The drawing under review shows one solid part. Ordinate dimensions are in mm from its lowest x, y, z. A direction names the side the tool comes from. Coordinates: 2 decimals unless noted, no trailing zeros. Order: outer loops, then holes, each group sorted by start corner. A loop starts at its lowest first (then second) coordinate and runs counter-clockwise, first axis right, second up. Notation, with made-up numbers: (64, 36.5) -> (78, 36.5) arc R16 cw to (78, 41.5) -> close; hole circle Ø3 at (-19, 86.5). An arc over 180 degrees is marked (long way). Write item = value, one per line.
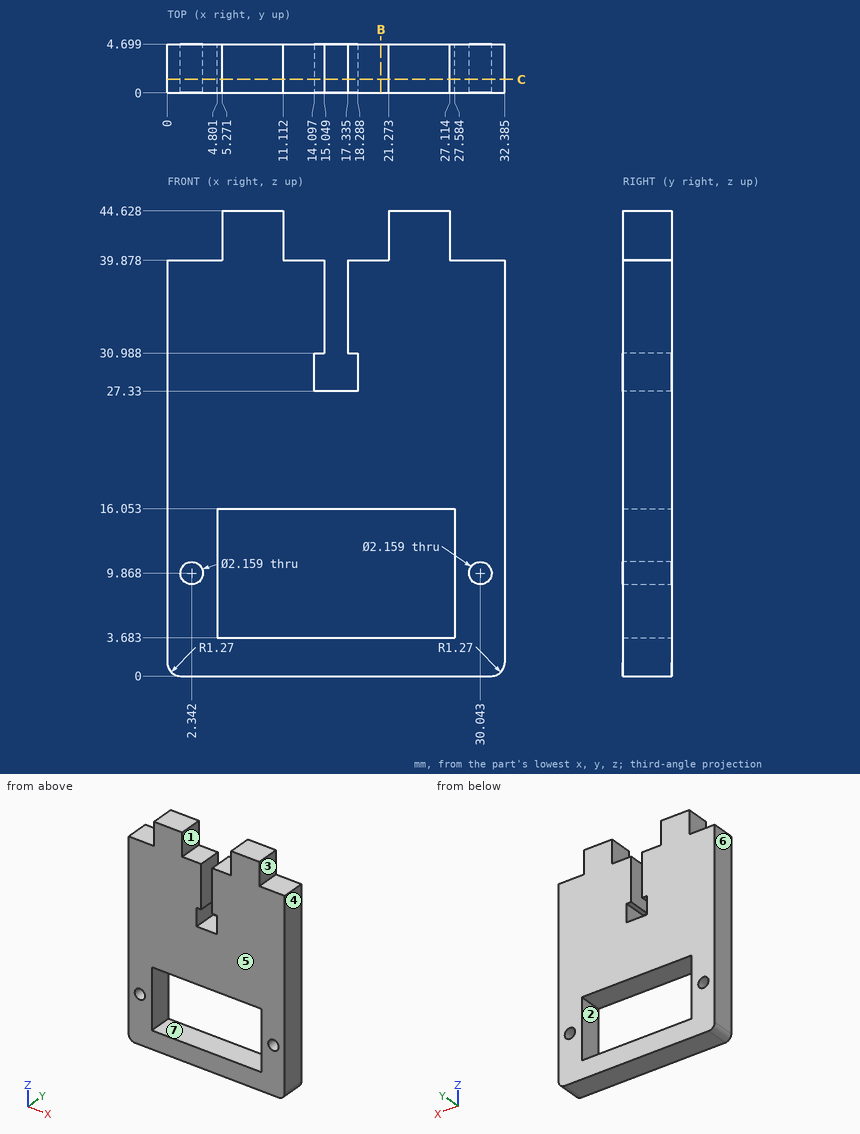
(1) For the marked faces 1, 2, 3 and 4, list the 3-axis set-ups (+Z, -Z, +X, -X, +Y, -Y) from which the entire face can be reached by the end or side of a thin tool; tool diameter is ignored.
Report:
face_1 = +Z, +Y, -Y
face_2 = +Y, -Y
face_3 = +Z, +X, +Y, -Y
face_4 = +Z, -Z, +X, +Y, -Y
(2) Insertion check: pin 1 (1.3 mm diameter, centred on x = 15.5, y = 3.5, fed in from +Z); pin 2 (1.9 mm diameter, centred on x = 30.04, z = 9.87, fed in from -Y). Each pin has a flat end and moves straight along its axis. Give the tip position at first contact, or say it passes through.
Report:
pin_1 = 39.88
pin_2 = through
(3) For L1, parallel to X at y = 1.05, z = 29 (1 decimal); L2, parallel to X at y = 3.1, z = 43.5 (1 decimal); L3, parallel to Z at x = 13.5, y = 3.5, list the stretches that pass through material, from the lowest coordinate up.
Report:
L1 = 0 to 14.1, 18.3 to 32.4
L2 = 5.3 to 11.1, 21.3 to 27.1
L3 = 0 to 3.68, 16.05 to 39.88
(4) We need section C-C (y = 1.3). Give the number of separate pieces and of enclosed holes in the cut face, and give its area (3 significant figures).
Report:
separate_pieces = 1
enclosed_holes = 3
area = 1,020 mm²
(5) The part is to be moulded in two halves that separate along X. For the marked faces 5, 6 and 7, say which applies: released by +X, released by -X, zero draft, split by the parting line, or undercut.
Report:
face_5 = zero draft
face_6 = released by -X
face_7 = undercut
(6) We need section B-B (x = 20.5). Write out the cut boundary in (y, z), and give its area (3 significant figures).
Report:
outline = (0, 0) -> (4.7, 0) -> (4.7, 3.68) -> (0, 3.68) -> close; (0, 16.05) -> (4.7, 16.05) -> (4.7, 39.88) -> (0, 39.88) -> close
area = 129 mm²
